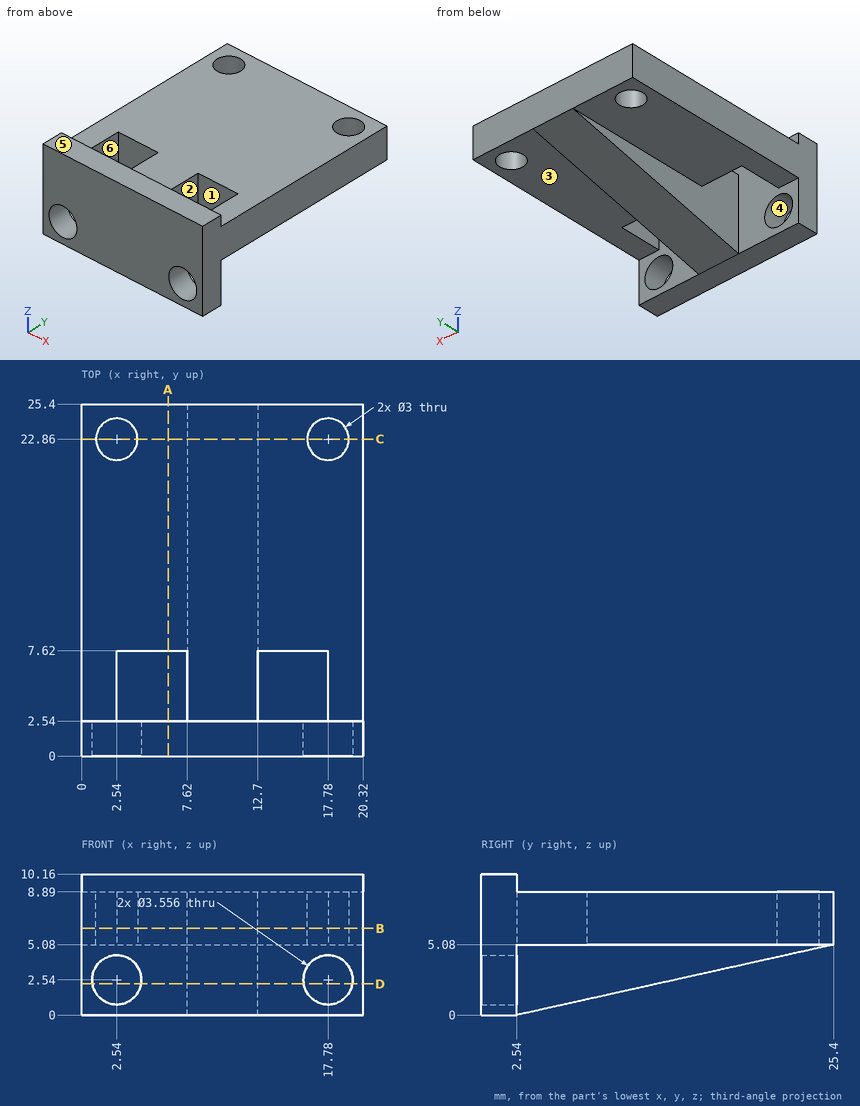
Here's the drawing with two shaded views (mm, measured from the low corner). I have some questions. A direction names the side the tool comes from. Coordinates: 2 decimals unless noted, no trailing zeros. Write each loop counter-clockwise with the first axis right and the second up, starting at its lowest first coordinate (ties: lowest second). Pieces come first, ordered by that corner, then holes.
Item 1: If we mould it in two halves opening along Z, with no side actions, what happens to the marked faces 4, 5 and 6? For each: +Z half, -Z half, draft (parallel to the pull), parting line (faces both ways), or undercut.
Item 2: I want a section at D-D on z = 2.25. Write out the boundary of the cut face in (x, y) (3 decimals).
Item 3: If I drill on line 1 (X direction, y = 1.55, z = 2.54); line 2 (Z direction, x = 15.25, y = 16.5); line 3 (Y direction, x = 13, z = 6.5), over which ranges is the centre line in solid material (lowest first)?
Item 4: I want a section at B-B on z = 6.25. Write out the boundary of the cut face in (x, y).
Item 5: Will these pins go through, and if not, where does the flat tip stop? pin 1 (3 mm diameter, centred on x = 17.78, z = 2.54, fed in from -Y); pin 2 (5 mm diameter, centred on x = 2.54, y = 22.86, fed in from +Z); pin 3 (3 mm diameter, centred on x = 6.5, z = 5, fed in from +Y); pin 4 (4 mm diameter, centred on x = 18, y = 16.5, fed in from -Z).
Item 6: I want a section at C-C on y = 22.86. Write out the boundary of the cut face in (x, z), and give its area (3 significant figures).
Item 7: On a 3-axis mill with a long thin cutter (end or side, diameter ignored), from which of +Z, -Z, +X, -X, +Y, -Y can I reach the whole of each face in a straight line? I mean the marked faces 1, 2 and 3. Say none if no direction works.
Item 8: I want a section at A-A on x = 6.25. Write out the boundary of the cut face in (y, z).
Findings below:
1. face 4: undercut
1. face 5: +Z half
1. face 6: draft
2. outline: (0, 0) - (0.786, 0) - (0.786, 2.54) - (0, 2.54) - close; (4.294, 0) - (16.026, 0) - (16.026, 2.54) - (12.7, 2.54) - (12.7, 12.665) - (7.62, 12.665) - (7.62, 2.54) - (4.294, 2.54) - close; (19.534, 0) - (20.32, 0) - (20.32, 2.54) - (19.534, 2.54) - close
3. line 1: x = 0 to 0.76, 4.32 to 16, 19.56 to 20.32
3. line 2: z = 5.08 to 8.89
3. line 3: y = 0 to 2.54, 7.62 to 25.4
4. outline: (0, 0) - (20.32, 0) - (20.32, 25.4) - (0, 25.4) - close; hole circle Ø3 at (2.54, 22.86); hole (2.54, 2.54) - (7.62, 2.54) - (7.62, 7.62) - (2.54, 7.62) - close; hole (12.7, 2.54) - (17.78, 2.54) - (17.78, 7.62) - (12.7, 7.62) - close; hole circle Ø3 at (17.78, 22.86)
5. pin 1: passes through
5. pin 2: stops at z = 8.89
5. pin 3: stops at y = 25.4
5. pin 4: stops at z = 5.08
6. outline: (0, 5.08) - (1.04, 5.08) - (1.04, 8.89) - (0, 8.89) - close; (4.04, 5.08) - (7.62, 5.08) - (7.62, 4.52) - (12.7, 4.52) - (12.7, 5.08) - (16.28, 5.08) - (16.28, 8.89) - (4.04, 8.89) - close; (19.28, 5.08) - (20.32, 5.08) - (20.32, 8.89) - (19.28, 8.89) - close
6. area: 57.4 mm2
7. face 1: +Z, -Z
7. face 2: -Z
7. face 3: -Z, +X, +Y
8. outline: (0, 0) - (2.54, 0) - (2.54, 10.16) - (0, 10.16) - close; (7.62, 5.08) - (25.4, 5.08) - (25.4, 8.89) - (7.62, 8.89) - close
